from build123d import *

# Parameters (mm, degrees)
SKETCH_2_R          = 1.4
CUT_EXTRUDE_1_DEPTH = 10
SKETCH_3_R          = 0.25
EXTRUDE_1_DEPTH     = 20
SKETCH_4_R          = 0.25
EXTRUDE_2_DEPTH     = 20


with BuildPart() as part:
    # 草图1 → 旋转1 (revolve)
    with BuildSketch(Plane.XY):
        Polygon((0, 40.1), (-16, 40.1), (-16, 38.1), (-7.75, 38.1), (-7.75, 6), (-2.95, 6), (-2.95, 0), (0, 0), align=None)
    revolve(axis=Axis((0, 0, 0), (0, 1, 0)))

    # 草图2 → 切除-拉伸1 (cut)
    with BuildSketch(Plane(origin=(0, 40.1, 0), x_dir=(1, 0, 0), z_dir=(0, 1, 0))):
        with Locations((0, 12.5)):
            Circle(SKETCH_2_R)
        with Locations((10.825317547, -6.25)):
            Circle(SKETCH_2_R)
        with Locations((-10.825317547, -6.25)):
            Circle(SKETCH_2_R)
    extrude(amount=-CUT_EXTRUDE_1_DEPTH, mode=Mode.SUBTRACT)

    # 草图3 → 凸台-拉伸1 (add)
    with BuildSketch(Plane(origin=(0, 40.1, 0), x_dir=(1, 0, 0), z_dir=(0, 1, 0))):
        with Locations((-6.5, 0)):
            Circle(SKETCH_3_R)
        with Locations((6.5, 0)):
            Circle(SKETCH_3_R)
        with Locations((-6.470567497, 0.617864281)):
            Circle(SKETCH_3_R)
        with Locations((6.470567497, -0.617864281)):
            Circle(SKETCH_3_R)
        with Locations((-6.382536532, 1.230133088)):
            Circle(SKETCH_3_R)
        with Locations((6.382536532, -1.230133088)):
            Circle(SKETCH_3_R)
        with Locations((-6.236704328, 1.831261619)):
            Circle(SKETCH_3_R)
        with Locations((6.236704328, -1.831261619)):
            Circle(SKETCH_3_R)
        with Locations((-6.034391565, 2.415805962)):
            Circle(SKETCH_3_R)
        with Locations((6.034391565, -2.415805962)):
            Circle(SKETCH_3_R)
        with Locations((-5.777430416, 2.978472391)):
            Circle(SKETCH_3_R)
        with Locations((5.777430416, -2.978472391)):
            Circle(SKETCH_3_R)
        with Locations((-5.468147963, 3.514165313)):
            Circle(SKETCH_3_R)
        with Locations((5.468147963, -3.514165313)):
            Circle(SKETCH_3_R)
        with Locations((-5.109345116, 4.01803341)):
            Circle(SKETCH_3_R)
        with Locations((5.109345116, -4.01803341)):
            Circle(SKETCH_3_R)
        with Locations((-4.704271248, 4.485513575)):
            Circle(SKETCH_3_R)
        with Locations((4.704271248, -4.485513575)):
            Circle(SKETCH_3_R)
        with Locations((-4.256594771, 4.912372233)):
            Circle(SKETCH_3_R)
        with Locations((4.256594771, -4.912372233)):
            Circle(SKETCH_3_R)
        with Locations((-3.770369912, 5.294743688)):
            Circle(SKETCH_3_R)
        with Locations((3.770369912, -5.294743688)):
            Circle(SKETCH_3_R)
        with Locations((-3.25, 5.629165125)):
            Circle(SKETCH_3_R)
        with Locations((3.25, -5.629165125)):
            Circle(SKETCH_3_R)
    extrude(amount=EXTRUDE_1_DEPTH)

    # 草图4 → 凸台-拉伸2 (add)
    with BuildSketch(Plane.XZ):
        with Locations((0, -2.5)):
            Circle(SKETCH_4_R)
        with Locations((-0.647047613, -2.414814566)):
            Circle(SKETCH_4_R)
        with Locations((-1.25, -2.165063509)):
            Circle(SKETCH_4_R)
        with Locations((-1.767766953, -1.767766953)):
            Circle(SKETCH_4_R)
        with Locations((-2.165063509, -1.25)):
            Circle(SKETCH_4_R)
        with Locations((-2.414814566, -0.647047613)):
            Circle(SKETCH_4_R)
        with Locations((-2.5, 0)):
            Circle(SKETCH_4_R)
        with Locations((-2.414814566, 0.647047613)):
            Circle(SKETCH_4_R)
        with Locations((-2.165063509, 1.25)):
            Circle(SKETCH_4_R)
        with Locations((-1.767766953, 1.767766953)):
            Circle(SKETCH_4_R)
        with Locations((-1.25, 2.165063509)):
            Circle(SKETCH_4_R)
        with Locations((-0.647047613, 2.414814566)):
            Circle(SKETCH_4_R)
        with Locations((0, 2.5)):
            Circle(SKETCH_4_R)
        with Locations((0.647047613, 2.414814566)):
            Circle(SKETCH_4_R)
        with Locations((1.25, 2.165063509)):
            Circle(SKETCH_4_R)
        with Locations((1.767766953, 1.767766953)):
            Circle(SKETCH_4_R)
        with Locations((2.165063509, 1.25)):
            Circle(SKETCH_4_R)
        with Locations((2.414814566, 0.647047613)):
            Circle(SKETCH_4_R)
        with Locations((2.5, 0)):
            Circle(SKETCH_4_R)
        with Locations((2.414814566, -0.647047613)):
            Circle(SKETCH_4_R)
        with Locations((2.165063509, -1.25)):
            Circle(SKETCH_4_R)
        with Locations((1.767766953, -1.767766953)):
            Circle(SKETCH_4_R)
        with Locations((1.25, -2.165063509)):
            Circle(SKETCH_4_R)
        with Locations((0.647047613, -2.414814566)):
            Circle(SKETCH_4_R)
    extrude(amount=EXTRUDE_2_DEPTH)


solid = part.part
Model file for the job. Use its own axes, mm. A direction names the side the tool comes from. Give positions to 0.01 mm unless a question says otherwise; leave off trailing zeros. Loops run counter-clockwise (first coordinate to the right, second up) from the corner with the lowest first, then second, coordinate; pieces in that order, holes last.
Item 1: Drop flat-ended pins along their axis: P1, Ø4, axis at x = -11, z = -2, coming from the +Y side; P2, Ø3, axis at y = 42.5, z = -11, coming from the -X side; P3, Ø12, axis at x = -7, y = 19.5, coming from the -Z side; P4, Ø1.5, axis at x = -4, y = 52, coming from the -Z side. Give the stop position or say it passes through.
Check values:
P1: stops at y = 40.1
P2: passes through
P3: stops at z = -7.69
P4: stops at z = -5.88
Item 2: Mould opens along X. For faces 1 (the face through (12.16, 39.11, 5.83)), 2 (the face through (4, 38.1, -7)), 3 (the face through (3.47, 39.09, -15.62)) say: +X half, -X half, draft (parallel to the pull), parting line (faces both ways), or undercut.
Check values:
face 1: undercut
face 2: draft
face 3: parting line
Item 3: Which spindle directions (+Z, -Z, +X, -X, +Y, -Y) get a long thin tool onto all of the face, cutting with end or side? Do faces 4 (the face through (0.75, 39.11, -13.68)), 5 (the face through (0, 40.1, 0)), 6 (the face through (2.947, 2.958, 0.13)). Say none if no direction does.
Check values:
face 4: +Y, -Y
face 5: +Y
face 6: -Y
Item 4: Slice it at B-B (z = -10). Write the cut outline in (x, y).
Check values:
outline: (-12.49, 38.1) - (12.49, 38.1) - (12.49, 40.1) - (-12.49, 40.1) - close
Item 5: Slice it at A-A (y = -5). Give the number of separate pieces and of enclosed holes in the cut face, plus the area to 3 significant figures.
Check values:
separate pieces: 24
enclosed holes: 0
area: 4.71 mm2
Item 6: Drill centre lines: line 1 along X through (y, z) = (38.6, 6.25); line 2 along Y through (x, z) = (-4, 7); line 3 along Z through (x, y) = (0, 38.6). Where is each one in solid material? Low to high.
Check values:
line 1: x = -14.73 to -12.23, -9.43 to 9.43, 12.23 to 14.73
line 2: y = 38.1 to 40.1
line 3: z = -16 to -13.9, -11.1 to 16
Item 7: Slice it at D-D (z = 13). Write the cut outline in (x, y), plus the area to 3 significant figures.
Check values:
outline: (-9.33, 38.1) - (9.33, 38.1) - (9.33, 40.1) - (-9.33, 40.1) - close
area: 37.3 mm2
Item 8: Slice it at C-C (y = 26). Write the cut outline in (x, z), plus the area to 3 significant figures.
Check values:
outline: circle Ø15.5 at (0, 0)
area: 189 mm2
